Verification items for the finished model (mm, model axes). A direction names the side the tool comes from. Round coordinates to 2 decimals unless told otherwise and drop trailing zeros. Write each loop counter-clockwise with the first axis right and the second up, starting at its lowest first coordinate (ties: lowest second). Pieces come first, ordered by that corner, then holes. Notation, with made-up numbers: (54, 26) -> (75, 26) arc R27 ccw to (75, 47) -> close; hole circle Ø8 at (-36, 19). An arc over 180 degrees is marked (long way). Answer as a JSON object with one key per item and string values. Group by question number.
(1) Sectioned sample at B-B on z = 0. Record the cut outline in (x, y), and give its area (3 significant figures).
(2) Sectioned sample at A-A on y = 15. Record the cut outline in (x, z), and give its area (3 significant figures).
(3) Scan lines: L1, parallel to X at y = 15.9, z = 0; L2, parallel to X at y = 4.5, z = 0; L3, parallel to X at y = -0.85, z = -7.3. Record each from-to range of solid material in increasing order. Write a range as from..to.
(4) Set-up check for faces 5 (the face through (0, 15.8, 0)), 6 (the face through (12, 1.5, 6)), 7 (the face through (-7.33, -0.74, -5.8)), 8 (the face through (10, 1, 8)): record each of +Z, -Z, +X, -X, +Y, -Y from which the full face is reachable in a straight line by a thin tool's end or side.
(5) Sectioned sample at C-C on x = 23.2. Record the cut outline in (y, z).
(6) Draft check along X on faces 1 (the face through (33.1, -1, 0)), 2 (the face through (11, -1.5, 0)), 3 (the face through (-9.9, -1, 0)), 4 (the face through (13, 0.76, 4.37)). Enter one of: released by +X, released by -X, zero draft, split by the parting line, or undercut.
(7) Gauge pin test, flat ends, axial feed: pin 1 Ø2 at (y, z) = (4.5, -1) entering from +X; pin 2 Ø0.5 at (y, z) = (0.5, 6.5) entering from +X; pin 3 Ø4.5 at (x, z) = (12, 7) entering from +Y. Record the tip position at first contact, or that the pin passes through.
```python
from build123d import *

# Parameters (mm, degrees)
SKETCH1_R          = 8.1
EXTRUDE1_DEPTH     = 16
EXTRUDE1_2_DEPTH   = 16
FILLET1_R          = 0.5
SKETCH2_R          = 6.6
CUT_EXTRUDE2_DEPTH = 0.2
FILLET2_R          = 0.5
SKETCH3_W          = 43
SKETCH3_H          = 19.6
SKETCH3_R          = 1.5
EXTRUDE2_DEPTH     = 1.5
SKETCH4_W          = 2
SKETCH4_H          = 5
EXTRUDE3_DEPTH     = 1.5
FILLET3_R          = 2


with BuildPart() as part:
    # Sketch1 → Extrude1 (new body)
    with BuildSketch(Plane(origin=(0, 0, 0), x_dir=(1, 0, 0), z_dir=(0, 1, 0))):
        with Locations(Location((0, 0, 0), (0, 0, 270))):
            Circle(SKETCH1_R)
    extrude(amount=EXTRUDE1_DEPTH)

    # Fillet1
    fillet1_edges = [part.edges().sort_by_distance(p)[0] for p in [
        (0, 0, -8.1),
        (0, 16, -8.1),
    ]]
    fillet(fillet1_edges, radius=FILLET1_R)


with BuildPart() as body_2:
    # Sketch1 → Extrude1 2 (new body)
    with BuildSketch(Plane(origin=(0, 0, 0), x_dir=(1, 0, 0), z_dir=(0, 1, 0))):
        with Locations(Location((23.2, 0, 0), (0, 0, 270))):
            Circle(SKETCH1_R)
    extrude(amount=EXTRUDE1_2_DEPTH)


with BuildPart() as cut_extrude2_tool:
    # Sketch2 → Cut-Extrude2 (new body)
    with BuildSketch(Plane(origin=(0, 16, 0), x_dir=(-1, 0, 0), z_dir=(0, 1, 0))):
        with Locations(Location((-23.2, 0, 0), (0, 0, 90))):
            Circle(SKETCH2_R)
        with Locations(Location((0, 0, 0), (0, 0, 90))):
            Circle(SKETCH2_R)
    extrude(amount=-CUT_EXTRUDE2_DEPTH)


with BuildPart() as part_1:
    add(part.part)

    # Cut-Extrude2: cut by cut_extrude2_tool
    add(cut_extrude2_tool.part, mode=Mode.SUBTRACT)



with BuildPart() as body_2_1:
    add(body_2.part)

    # Cut-Extrude2: cut by cut_extrude2_tool
    add(cut_extrude2_tool.part, mode=Mode.SUBTRACT)

    # Fillet2
    fillet2_edges = [body_2_1.edges().sort_by_distance(p)[0] for p in [
        (23.2, 0, -8.1),
        (23.2, 16, -8.1),
    ]]
    fillet(fillet2_edges, radius=FILLET2_R)


with BuildPart() as part_2:
    add(part_1.part)

    add(body_2_1.part)  # Extrude2 merges body 2
    # Sketch3 → Extrude2 (add)
    with BuildSketch(Plane.XZ):
        with Locations((11.6, 0)):
            Rectangle(SKETCH3_W, SKETCH3_H)
        with Locations(Location((-7.4, -7.3, 0), (0, 0, 270))):
            Circle(SKETCH3_R, mode=Mode.SUBTRACT)
        with Locations(Location((30.6, 7.3, 0), (0, 0, 270))):
            Circle(SKETCH3_R, mode=Mode.SUBTRACT)
    extrude(amount=EXTRUDE2_DEPTH)

    # Sketch4 → Extrude3 (add)
    with BuildSketch(Plane(origin=(0, 0, 0), x_dir=(-1, 0, 0), z_dir=(0, 1, 0))):
        with Locations((-10.6, 6.3)):
            Rectangle(SKETCH4_W, SKETCH4_H)
        with Locations((-12.6, 6.3)):
            Rectangle(SKETCH4_W, SKETCH4_H)
    extrude(amount=EXTRUDE3_DEPTH)

    # Fillet3
    fillet3_edges = [part_2.edges().sort_by_distance(p)[0] for p in [
        (9.6, 0.75, 3.8),
        (13.6, 0.75, 3.8),
        (9.6, 0.75, 8.8),
        (13.6, 0.75, 8.8),
    ]]
    fillet(fillet3_edges, radius=FILLET3_R - 0.0001)  # a hair under: the kernel refuses the full size


solid = part_2.part
```
Computed values:
{
 "1": {"outline": "(-9.9, -1.5) -> (33.1, -1.5) -> (33.1, 0) -> (30.8, 0) arc R0.5 ccw to (31.3, 0.5) -> (31.3, 15.5) arc R0.5 ccw to (30.8, 16) -> (29.8, 16) -> (29.8, 15.8) -> (16.6, 15.8) -> (16.6, 16) -> (15.6, 16) arc R0.5 ccw to (15.1, 15.5) -> (15.1, 0.5) arc R0.5 ccw to (15.6, 0) -> (7.6, 0) arc R0.5 ccw to (8.1, 0.5) -> (8.1, 15.5) arc R0.5 ccw to (7.6, 16) -> (6.6, 16) -> (6.6, 15.8) -> (-6.6, 15.8) -> (-6.6, 16) -> (-7.6, 16) arc R0.5 ccw to (-8.1, 15.5) -> (-8.1, 0.5) arc R0.5 ccw to (-7.6, 0) -> (-9.9, 0) -> close", "area": "577 mm2"},
 "2": {"outline": "circle Ø16.2 at (0, 0); circle Ø16.2 at (23.2, 0)", "area": "412 mm2"},
 "3": {"L1": "-7.9..-6.6, 6.6..7.9, 15.3..16.6, 29.8..31.1", "L2": "-8.1..8.1, 15.1..31.3", "L3": "-9.9..-8.9, -5.9..33.1"},
 "4": {"face 5": "+Y", "face 6": "+Z, -Z, +Y", "face 7": "+Y, -Y", "face 8": "+Z, +Y"},
 "5": {"outline": "(-1.5, -9.8) -> (0, -9.8) -> (0, -7.6) arc R0.5 ccw to (0.5, -8.1) -> (15.5, -8.1) arc R0.5 ccw to (16, -7.6) -> (16, -6.6) -> (15.8, -6.6) -> (15.8, 6.6) -> (16, 6.6) -> (16, 7.6) arc R0.5 ccw to (15.5, 8.1) -> (0.5, 8.1) arc R0.5 ccw to (0, 7.6) -> (0, 9.8) -> (-1.5, 9.8) -> close"},
 "6": {"face 1": "released by +X", "face 2": "zero draft", "face 3": "released by -X", "face 4": "undercut"},
 "7": {"pin 1": "x = 31.3", "pin 2": "x = 28.35", "pin 3": "y = 1.5"}
}
